Input: dimensioned drawing with shaded views. Units: mm. Origin: part minimum x, y, z. A direction names the side the tool comes from. Give positions to 0.01 mm unless a question says otherwise; leave off trailing zeros. Use CSV: the item, a comma, the result in double quotes.
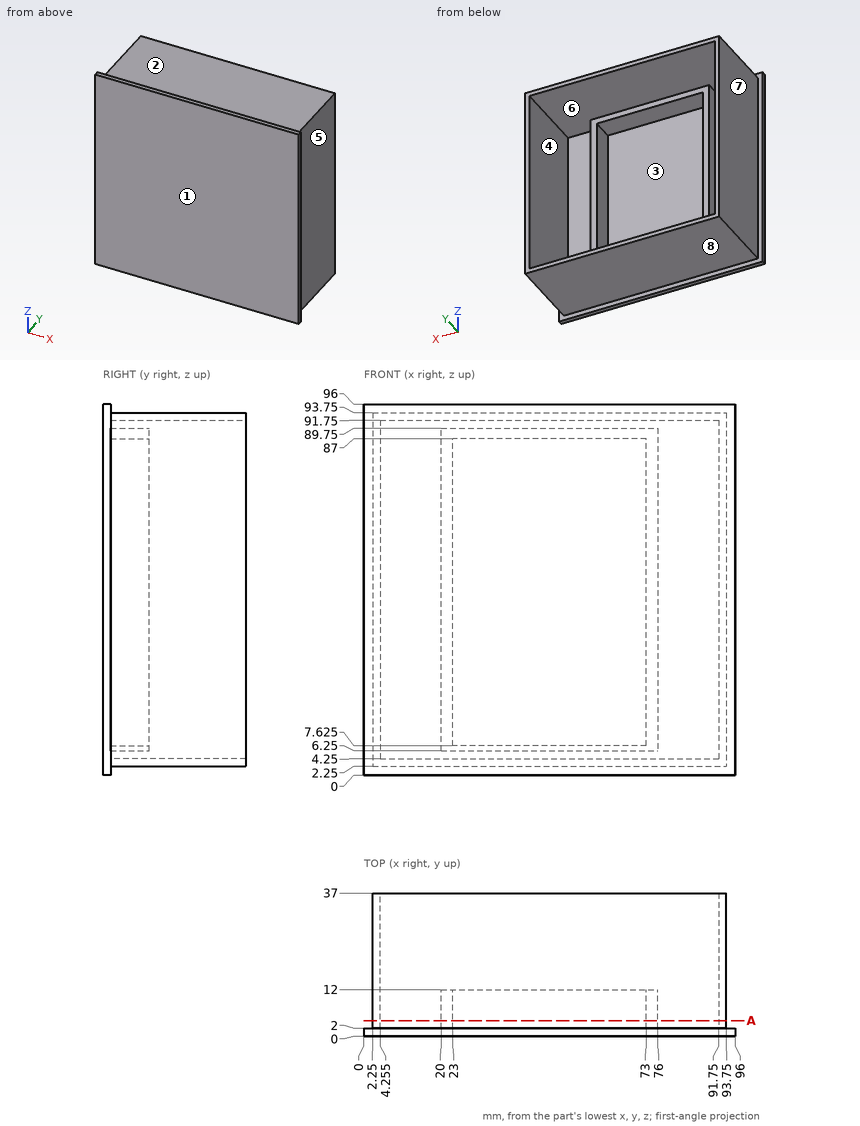
1. Access query for the marked faces 5, 6, 7 and 8. Directions: +Z, -Z, +X, -X, +Y, -Y. A direction counts if a zero-diameter tool reaches every point of the face in a straight line with its end or side. Return the directions, or none.
Answer below:
face 5,"+Z, -Z, +X, +Y"
face 6,"+Y"
face 7,"+Z, -Z, -X, +Y"
face 8,"-Z, +X, -X, +Y"
2. Pin query (flat end, axial travel): P1, Ø1, axis at x = 26, z = 45, coming from the +Y side; P2, Ø8, axis at x = 61.5, y = 6.5, coming from the +Z side; P3, Ø12, axis at y = 21, z = 63, coming from the -X side. Return the tip coordinate at first contact, or that it passes through.
Answer below:
P1,"stops at y = 2"
P2,"stops at z = 93.75"
P3,"stops at x = 2.25"
3. Ray query, line 1 along Z through (x, y) = (32, 31); line 2 along Y through (x, z) = (79.5, 91). Return the intervals inside material, ascending.
Answer below:
line 1,"z = 2.25 to 4.25, 91.75 to 93.75"
line 2,"y = 0 to 2"
4. Section query A-A on y = 4. Count the separate pieces of the cut face and the enclosed holes in it, plus the area to 3 significant figures.
Answer below:
separate pieces,"2"
enclosed holes,"2"
area,"1,420 mm²"
5. Mould query, pull axis Z, two halves, no side actions, for the marked faces 1, 2, 3 and 4. Classes: released by +Z, released by -Z, zero draft, split by the parting line, or undercut.
Answer below:
face 1,"zero draft"
face 2,"released by +Z"
face 3,"undercut"
face 4,"undercut"
